Autodesk Inventor part; units mm, degrees
ref_plane "Work Plane1" through (0, 0, -15) normal (0, 0, 1) x (1, 0, 0)
ref_plane "YZ Plane" through (0, 0, 0) normal (1, 0, 0) x (0, 1, 0)
ref_plane "XZ Plane" through (0, 0, 0) normal (0, 1, 0) x (-1, 0, 0)
sketch "Sketch1" plane through (0, 0, 0) normal (0, 0, 1) x (1, 0, 0)
  line L0 (0, 0) -> (25, 0)
  line L1 (25, 0) -> (25, 40)
  line L2 (25, 40) -> (0, 40)
  line L3 (0, 40) -> (0, 0)
  dimension "d1" = 25
  dimension "d2" = 40
  dimension "d3" = 25
extrude "Extrusion1" add sketch "Sketch1" against normal blind 30
sketch "Sketch2" plane through (25, 0, 0) normal (1, 0, 0) x (0, 0, -1)
  line L0 (0, 0) -> (30, 0)
  circle A0 centre (15, 6.56) radius 2.46
extrude "Extrusion2" cut sketch "Sketch2" against normal blind 30
sketch "Sketch3" plane through (0, 0, 0) normal (-1, 0, 0) x (0, 0, 1)
  line L0 (0, 0) -> (-30, 0)
  line L1 (-25.05, 0) -> (-4.95, 0)
  line L2 (-4.95, 0) -> (-4.95, 33.12)
  line L3 (-4.95, 33.12) -> (-25.05, 33.12)
  line L4 (-25.05, 33.12) -> (-25.05, 0)
  dimension "d11" = 20.1
extrude "Extrusion3" cut sketch "Sketch3" against normal blind 20
sketch "Sketch4" plane through (0, 0, 0) normal (0, -1, 0) x (1, 0, 0)
  line L0 (20, -4.95) -> (20, -25.05)
  line L1 (20, -15) -> (25, -15)
  line L2 (25, 0) -> (25, -30)
  line L3 (20, -8.025) -> (25, -8.025)
  line L4 (25, -8.025) -> (25, -21.975)
  line L5 (25, -21.975) -> (20, -21.975)
  line L6 (20, -21.975) -> (20, -8.025)
  line L7 (20, -8.025) -> (25, -21.975) construction
  line L8 (25, -8.025) -> (20, -21.975) construction
  line L9 (25, -12.54) -> (25, -17.46)
  point P0 (0, 0)
  point P1 (22.5, -15)
  dimension "d14" = 13.95
extrude "Extrusion4" add sketch "Sketch4" along normal blind 15
sketch "Sketch5" plane through (20, 0, 0) normal (-1, 0, 0) x (0, 0, 1)
  circle A0 centre (-15, 6.56) radius 2.46
  circle A1 centre (-15, 6.56) radius 4.7025
  circle A2 centre (-15, 6.56) radius 2.46
  circle A3 centre (-15, 6.56) radius 2.46
  point P0 (0, 0)
  dimension "d17" = 9.405
extrude "Extrusion5" cut sketch "Sketch5" against normal blind 2.1
sketch "Sketch6" plane through (25, 0, 0) normal (1, 0, 0) x (0, 0, -1)
  circle A0 centre (15, 6.56) radius 4.7025
  line L0 (15, 6.56) -> (15, 23.56)
  circle A1 centre (15, 23.56) radius 2.46
  point P0 (0, 0)
  dimension "d20" = 17
  dimension "d21" = 4.92
extrude "Extrusion6" cut sketch "Sketch6" against normal blind 10 contours A1
sketch "Sketch7" plane through (20, 0, 0) normal (-1, 0, 0) x (0, 0, 1)
  circle A0 centre (-15, 23.56) radius 2.46
  circle A1 centre (-15, 23.56) radius 4.7025
  point P0 (0, 0)
  dimension "d24" = 9.405
extrude "Extrusion7" cut sketch "Sketch7" against normal blind 2.1
sketch "Sketch9" plane through (25, 0, 0) normal (1, 0, 0) x (0, 0, -1)
  circle A0 centre (15, 6.56) radius 2.46
  circle A1 centre (15, 6.56) radius 2.46
  circle A2 centre (15, 23.56) radius 2.46
  circle A3 centre (15, 23.56) radius 2.46
  line L0 (30, 40) -> (30, 0)
  line L1 (30, 0) -> (30, 40)
  line L2 (30, 40) -> (0, 40)
  line L3 (0, 40) -> (0, 0)
  line L4 (0, 0) -> (8.025, 0)
  line L5 (21.975, 0) -> (21.975, -15)
  line L6 (21.975, -15) -> (8.025, -15)
  line L7 (8.025, -15) -> (8.025, 0)
  line L8 (0, 0) -> (8.025, 0)
  line L9 (21.975, 0) -> (30, 0)
extrude "Extrusion8" add sketch "Sketch9" along normal blind 5
sketch "Sketch10" plane through (0, 40, 0) normal (0, 1, 0) x (1, 0, 0)
  line L0 (0, 30) -> (30, 30)
  line L1 (30, 0) -> (0, 0)
  line L2 (0, 30) -> (30, 30)
  line L3 (30, 30) -> (30, 0)
  line L4 (30, 0) -> (0, 0)
  line L5 (0, 0) -> (0, 30)
extrude "Extrusion9" add sketch "Sketch10" along normal blind 30
sketch "Sketch12" plane through (30, 0, 0) normal (1, 0, 0) x (0, 0, -1)
  circle A0 centre (15, 6.56) radius 2.46
  line L0 (15, 6.56) -> (15, 15.06)
  circle A1 centre (15, 15.06) radius 2.525
  point P0 (0, 0)
  dimension "d31" = 8.5
  dimension "d33" = 5.05
extrude "Extrusion10" cut sketch "Sketch12" against normal blind 30 contours A1
sketch "Sketch14" plane through (0, 0, 0) normal (0, 0, 1) x (1, 0, 0)
  line L0 (30, 70) -> (0, 70)
  line L1 (0, 100) -> (-8, 100)
  line L2 (30, 0) -> (30, 70)
  line L3 (30, 118) -> (30, 70)
  line L4 (30, 105) -> (30, 100)
  line L5 (0, 70) -> (30, 70)
  line L6 (0, 70) -> (0, 100)
  line L7 (30, 122.5) -> (30, 118)
  line L8 (30, 70) -> (30, 145)
  line L9 (-2, 157.5) -> (-8, 160)
  line L10 (-2, 102.5) -> (-8, 100)
  line L11 (4, 130) -> (-2, 102.5)
  line L12 (4, 130) -> (-2, 157.5)
  line L13 (-8, 160) -> (15, 160)
  line L14 (30, 145) -> (15, 160)
  point P0 (0, 0)
  dimension "d47" = 30
extrude "Extrusion12" add sketch "Sketch14" against normal blind 30
sketch "Sketch15" plane through (0, 0, -25.05) normal (-1, 0, 0) x (0, 0, 1)
  line L0 (0, 33.12) -> (20.1, 33.12)
  line L1 (20.1, 33.12) -> (20.1, 0)
  line L2 (0, 33.12) -> (20.1, 33.12)
  line L3 (20.1, 33.12) -> (20.1, 31.1)
  line L4 (20.1, 31.1) -> (0, 31.1)
  line L5 (0, 31.1) -> (0, 33.12)
  point P0 (25.05, 0)
  dimension "d57" = 2.02
extrude "Extrusion13" add sketch "Sketch15" against normal blind 20
sketch "Sketch27" plane through (0, 0, 0) normal (0, 0, 1) x (1, 0, 0)
  point P0 (0, 0)
sketch "Sketch28" plane through (0, 0, 0) normal (0, 0, 1) x (1, 0, 0)
  line L0 (0, 100) -> (-8, 100)
  line L1 (0, 100) -> (-8, 100)
  line L2 (-8, 100) -> (-2, 102.5)
  line L3 (-8, 100) -> (-2, 102.5)
  line L4 (-2, 102.5) -> (4, 130)
  line L5 (-2, 102.5) -> (4, 130)
  line L6 (4, 130) -> (-2, 157.5)
  line L7 (4, 130) -> (-2, 157.5)
  line L8 (-2, 157.5) -> (-8, 160)
  line L9 (-2, 157.5) -> (-8, 160)
  line L10 (-8, 160) -> (15, 160)
  line L11 (-8, 160) -> (15, 160)
  line L12 (15, 160) -> (30, 145)
  line L13 (15, 160) -> (30, 145)
  line L14 (30, 145) -> (30, 93)
  line L15 (30, 0) -> (30, 145)
  line L16 (30, 93) -> (0, 93)
  line L17 (0, 0) -> (0, 100)
  line L18 (0, 93) -> (0, 100)
  dimension "d98" = 52
extrude "Extrusion14" add sketch "Sketch28" along normal blind 15
ref_plane "Work Plane1" through (0, 0, -15) normal (0, 0, 1) x (1, 0, 0)
mirror "Mirror1" about plane through (0, 0, -15) normal (0, 0, 1) of "Extrusion14"
properties part number "55mm_x_60mm"
Input: part model. Units: mm. Frame: model coordinates. A direction names the side the tool comes from. Coordinates: 2 decimals unless noted, no trailing zeros. Loops run counter-clockwise (first coordinate to the right, second up) from the corner with the lowest first, then second, coordinate; pieces in that order, holes last. Notation, with made-up numbers: (37, -22.75) -> (88, -22.75) arc R27 ccw to (88, 5.25) -> close; hole circle Ø3 at (-7, -3.5). An arc over 180 degrees is marked (long way). One line per item, written item: value.
(1) Set-up query: faces 4 (the face through (22.1, 21.5, -13)), 5 (the face through (10, 31.1, -15)), 6 (the face through (0, 62, -15)), 7 (the face through (15, 47, -30)). Return all of +Z, -Z, +X, -X, +Y, -Y with unobstructed straight access to the full face (end or side cutting, diameter ignored); none if empty.
Answer below:
face 4: -X
face 5: -X, -Y
face 6: +Z, -Z, -X, -Y
face 7: -Z, +X, -X, -Y
(2) Cut plane A-A (z = -15). Give the number of separate pieces and of enclosed holes in the cut face, then the cut area to 3 significant figures.
Answer below:
separate pieces: 4
enclosed holes: 0
area: 4,020 mm2
(3) Cut plane C-C (x = 8.5). Output: boundary loops of the cut face in (y, z), then the cut area to 3 significant figures.
Answer below:
outline: (0, -30) -> (93, -30) -> (93, -45) -> (160, -45) -> (160, 15) -> (93, 15) -> (93, 0) -> (0, 0) -> (0, -4.95) -> (31.1, -4.95) -> (31.1, -25.05) -> (0, -25.05) -> close
area: 6,180 mm2
(4) Cut plane B-B (y = 23.56). Output: boundary loops of the cut face in (x, z).
Answer below:
outline: (0, -30) -> (30, -30) -> (30, -17.46) -> (22.1, -17.46) -> (22.1, -19.7) -> (20, -19.7) -> (20, -25.05) -> (0, -25.05) -> close; (0, -4.95) -> (20, -4.95) -> (20, -10.3) -> (22.1, -10.3) -> (22.1, -12.54) -> (30, -12.54) -> (30, 0) -> (0, 0) -> close
(5) Pin query (flat end, axial travel): pin 1 Ø2.5 at (x, z) = (-2.5, -5.5) entering from -Y; pin 2 Ø3 at (y, z) = (8.5, -14.5) entering from -X; pin 3 Ø10 at (y, z) = (72.5, -15) entering from -X; pin 4 Ø11 at (y, z) = (6.56, -15) entering from +X. Return the tip coordinate at first contact, or that it passes through.
Answer below:
pin 1: stops at y = 100
pin 2: stops at x = 22.1
pin 3: stops at x = 0
pin 4: stops at x = 30
(6) Cut plane D-D (z = -39). Output: boundary loops of the cut face in (x, y).
Answer below:
outline: (-8, 100) -> (0, 100) -> (0, 93) -> (30, 93) -> (30, 145) -> (15, 160) -> (-8, 160) -> (-2, 157.5) -> (4, 130) -> (-2, 102.5) -> close
(7) Draft query along Y for faces 1 (the face through (25.995, 24.502, -17.272)), 2 (the face through (25, -15, -15)), 3 (the face through (10, 15, -4.95)). Return one class per face: pulls with the +Y half, pulls with the -Y half, needs draft (parallel to the pull), parting line crosses it, or undercut.
Answer below:
face 1: undercut
face 2: pulls with the -Y half
face 3: needs draft
(8) Ray query, line 1 along Z through (x, y) = (28.5, 6.56); line 2 along Z through (x, y) = (0.5, 31); line 3 along Y through (x, z) = (20.5, -15) (1 decimal). Return the intervals inside material, ascending.
Answer below:
line 1: z = -30 to -17.46, -12.54 to 0
line 2: z = -30 to -25.05, -4.95 to 0
line 3: y = -15 to 1.9, 11.3 to 12.5, 17.6 to 18.9, 28.3 to 154.5
